Geometry check sheet. Reference: the model listing, model coordinates, mm. Give positions to 0.01 mm unless a question says otherwise; leave off trailing zeros. Loops run counter-clockwise (first coordinate to the right, second up) from the corner with the lowest first, then second, coordinate; pieces in that order, holes last.
1. Material ranges on L1, parallel to Z at x = 22.5, y = 0.75; L2, parallel to X at y = 0.8, z = -10.5; L3, parallel to X at y = 1.05, z = -9, recorded low to high.
2. Go/stop test with a flat-tipped pin: pin 1 Ø1.8 at (x, z) = (22.5, -10) entering from +Y. Record where the tip stops, or that it passes through.
3. Cross-section at A-A, the plane z = 5. Record the cut outline in (x, y), plus the area to 3 significant figures.
4. Cross-section at B-B, the plane x = -22.5. Record the cut outline in (y, z), plus the area to 3 significant figures.
5. Release check for a two-part mould opening along Z. For faces 1 (the cylindrical face through (21.3, 1, -10.9)), 2 (the flat face through (0, 0, 0)), 3 (the flat face through (0, 1, -17.5)) record: +Z half, -Z half, draft (parallel to the pull), parting line (faces both ways), or undercut.
from build123d import *

# Parameters (mm, degrees)
CROQUIS1_W              = 60
CROQUIS1_H              = 35
SALIENTE_EXTRUIR1_DEPTH = 2
CORTAR_EXTRUIR1_REACH   = 4
CROQUIS2_R              = 1.5


with BuildPart() as part:
    # Croquis1 → Saliente-Extruir1 (new body)
    with BuildSketch(Plane(origin=(0, 0, 0), x_dir=(1, 0, 0), z_dir=(0, 1, 0))):
        Rectangle(CROQUIS1_W, CROQUIS1_H)
    extrude(amount=SALIENTE_EXTRUIR1_DEPTH)

    # Croquis2 → Cortar-Extruir1 (cut, up to next)
    with BuildSketch(Plane.XZ, mode=Mode.PRIVATE) as cortar_extruir1_sk1:
        with Locations((22.5, -10)):
            Circle(CROQUIS2_R)
    cortar_extruir1_tool1 = extrude(cortar_extruir1_sk1.sketch, amount=-CORTAR_EXTRUIR1_REACH, mode=Mode.PRIVATE) & part.part
    add(cortar_extruir1_tool1.solids().sort_by_distance((22.5, 0, -10))[0], mode=Mode.SUBTRACT)
    # Croquis2 → Cortar-Extruir1 (cut, up to next)
    with BuildSketch(Plane.XZ, mode=Mode.PRIVATE) as cortar_extruir1_sk2:
        with Locations((22.5, 5)):
            Circle(CROQUIS2_R)
    cortar_extruir1_tool2 = extrude(cortar_extruir1_sk2.sketch, amount=-CORTAR_EXTRUIR1_REACH, mode=Mode.PRIVATE) & part.part
    add(cortar_extruir1_tool2.solids().sort_by_distance((22.5, 0, 5))[0], mode=Mode.SUBTRACT)
    # Croquis2 → Cortar-Extruir1 (cut, up to next)
    with BuildSketch(Plane.XZ, mode=Mode.PRIVATE) as cortar_extruir1_sk3:
        with Locations((-22.5, -10)):
            Circle(CROQUIS2_R)
    cortar_extruir1_tool3 = extrude(cortar_extruir1_sk3.sketch, amount=-CORTAR_EXTRUIR1_REACH, mode=Mode.PRIVATE) & part.part
    add(cortar_extruir1_tool3.solids().sort_by_distance((-22.5, 0, -10))[0], mode=Mode.SUBTRACT)
    # Croquis2 → Cortar-Extruir1 (cut, up to next)
    with BuildSketch(Plane.XZ, mode=Mode.PRIVATE) as cortar_extruir1_sk4:
        with Locations((-22.5, 5)):
            Circle(CROQUIS2_R)
    cortar_extruir1_tool4 = extrude(cortar_extruir1_sk4.sketch, amount=-CORTAR_EXTRUIR1_REACH, mode=Mode.PRIVATE) & part.part
    add(cortar_extruir1_tool4.solids().sort_by_distance((-22.5, 0, 5))[0], mode=Mode.SUBTRACT)


solid = part.part
Result:
1. L1: z = -17.5 to -11.5, -8.5 to 3.5, 6.5 to 17.5
1. L2: x = -30 to -23.91, -21.09 to 21.09, 23.91 to 30
1. L3: x = -30 to -23.62, -21.38 to 21.38, 23.62 to 30
2. pin 1: passes through
3. outline: (-30, 0) - (-24, 0) - (-24, 2) - (-30, 2) - close; (-21, 0) - (21, 0) - (21, 2) - (-21, 2) - close; (24, 0) - (30, 0) - (30, 2) - (24, 2) - close
3. area: 108 mm2
4. outline: (0, -17.5) - (2, -17.5) - (2, -11.5) - (0, -11.5) - close; (0, -8.5) - (2, -8.5) - (2, 3.5) - (0, 3.5) - close; (0, 6.5) - (2, 6.5) - (2, 17.5) - (0, 17.5) - close
4. area: 58.0 mm2
5. face 1: undercut
5. face 2: draft
5. face 3: -Z half
